from build123d import *

# Parameters (mm, degrees)
CIRPATTERN1_COUNT = 6


with BuildPart() as part:
    # Sketch2 → Revolve2 (revolve)
    with BuildSketch(Plane.XY, mode=Mode.PRIVATE) as revolve2_sk:
        Polygon((-20.32, 31.75), (-12.192, 26.67), (15.766051224, 26.67), (21.06299661, 21.373054614), (81.28, 38.1), (81.28, 44.45), (2.54, 44.45), (2.54, 40.64), (-1.27, 40.64), (-1.27, 44.45), (-7.62, 44.45), (-7.62, 41.529), (-10.668, 41.529), (-10.668, 34.417), (-17.78, 34.417), (-17.78, 41.529), (-20.32, 41.529), align=None)
    revolve(revolve2_sk.sketch.rotate(Axis((0, 0, 0), (1, 0, 0)), 90), axis=Axis((0, 0, 0), (1, 0, 0)))

    # Sketch4 → 1/2 (0.5) Diameter Hole1 (revolve, cut)
    with BuildSketch(Plane(origin=(21.06299661, 44.45, 0), x_dir=(0, 0, 1), z_dir=(1, 0, 0))):
        Polygon((0, 0), (0, 15.24), (6.35, 11.424535069), (6.35, 0), align=None)
    f_1_2_0_5_diameter_hole1 = revolve(axis=Axis((21.06299661, 50.8, 0), (0, -1, 0)), mode=Mode.SUBTRACT)

    # CirPattern1: 1/2 (0.5) Diameter Hole1 ×6 about axis
    cirpattern1_axis = Axis((0, 0, 0), (1, 0, 0))
    for i in range(1, CIRPATTERN1_COUNT):
        add(f_1_2_0_5_diameter_hole1.rotate(cirpattern1_axis, i * 360 / CIRPATTERN1_COUNT), mode=Mode.SUBTRACT)


solid = part.part
Build history of the part. All positions in model axes, mm. A direction names the side the tool comes from. Coordinates: 2 decimals unless noted, no trailing zeros. Write each loop counter-clockwise with the first axis right and the second up, starting at its lowest first coordinate (ties: lowest second). Pieces come first, ordered by that corner, then holes.
(1) Cut at C-C on x = 61. List the corners of the cut face in (y, z), and give its area (3 significant figures).
(2) Drill centre lines: line 1 (X direction, y = -21, z = 35.5); line 2 (X direction, y = -39.5, z = 0); line 3 (Y direction, x = 8.75, z = 0). Where is each one in solid material? Low to high.
(3) Cut at B-B on y = -36. State how many separate pieces and enclosed holes the cut face has, and give its area (3 significant figures).
(4) 3-axis set-ups, long thin cutter, end or side, ignore diameter. For faces 4 (the cylindrical face through (0.608, -40.294, -5.291)), 5 (the flat face through (-7.62, -40, -13)), 6 (the flat face through (81.28, -20, -33)), 7 (the cylindrical face through (14.767, 38.818, -0.827)): which of +Z, -Z, +X, -X, +Y, -Y reach the whole face in a straight line?
(5) Mould opens along Y. For faces 1 (the cylindrical face through (1.983, -26.443, -3.472)), 2 (the cylindrical face through (14.767, -38.818, 0.827)), 3 (the cylindrical face through (41.4, -30, -32.8)) say: pulls with the +Y half, pulls with the -Y half, needs draft (parallel to the pull), parting line crosses it, or undercut.
(6) Pin check, flat tips, straight feed: pin 1 Ø12 at (x, z) = (10.5, -17.5) entering from +Y; pin 2 Ø1 at (x, z) = (28.5, 20) entering from +Y; pin 3 Ø3 at (x, z) = (22.5, -31) entering from -Y. Stop position of each tip, or through.
Working result:
1. outline: circle Ø88.9 at (0, 0); hole circle Ø64.93 at (0, 0)
1. area: 2,900 mm2
2. line 1: x = -20.32 to -17.78, -10.67 to -1.27, 2.54 to 14.73, 27.4 to 81.28
2. line 2: x = -20.32 to -17.78, -10.67 to 14.71, 27.41 to 81.28
2. line 3: y = -44.45 to -26.67, 26.67 to 44.45
3. separate pieces: 2
3. enclosed holes: 1
3. area: 4,560 mm2
4. face 4: none
4. face 5: -X
4. face 6: +Z, -Z, +X, +Y, -Y
4. face 7: +Y
5. face 1: undercut
5. face 2: needs draft
5. face 3: parting line crosses it
6. pin 1: stops at y = 42.94
6. pin 2: stops at y = 39.94
6. pin 3: stops at y = -33.25
